Check sheet for the modelled part. Datum: model origin and axes. Units: mm. Face numbers are marked on the shaded views. A direction names the side the tool comes from. Give positions to 0.01 mm unless a question says otherwise; leave off trailing zeros. Order: outer loops, then holes, each group sorted by start corner. A loop starts at its lowest first (then second) coordinate and runs counter-clockwise, first axis right, second up. Notation, with made-up numbers: (44, -22) -> (61, -22) arc R29 ccw to (61, 10) -> close; hole circle Ø4 at (46.5, 51). An arc over 180 degrees is marked (long way). Answer in a Markdown table with one row per item. Add a question column.
(1) Thickness scan on L1, parallel to Z at x = -22, y = 269; L2, parallel to X at y = 117.5, z = -7.5; L3, parallel to Z at x = 4, y = 8. Record the ranges inside material, lowest first. Write a range as [from, to].
(2) Cross-section at D-D (y = 2). Record the cut outline in (x, z).
(3) Cross-section at B-B (x = 5). Record the cut outline in (y, z).
(4) Cross-section at C-C (y = 521.5). Record the cut outline in (x, z), then the cut area to 3 significant figures.
(5) Release check for a two-part mould opening along Z. For the marked faces 1, 2, 3 and 4 record: released by +Z, released by -Z, zero draft, split by the parting line, or undercut.
(6) Cross-section at A-A (z = 10). Record the cut outline in (x, y).
(7) Set-up check for the marked faces 5 and 6: record each of +Z, -Z, +X, -X, +Y, -Y from which the full face is reachable in a straight line by a thin tool's end or side.
(8) Go/stop test with a flat-tipped pin: pin 1 (1.5 mm diameter, centred on x = 29, y = -6.5, fed in from -Z). Record where the tip stops, or that it passes through.
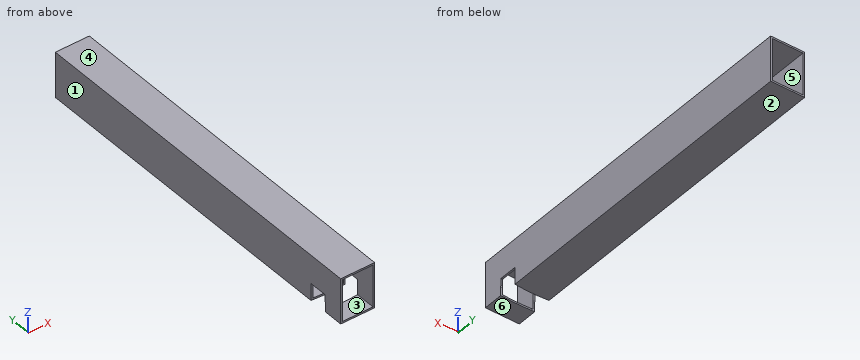
```python
from build123d import *

# Parameters (mm, degrees)
F0_W          = 60
F0_H          = 80
F0_W_2        = 54
F0_H_2        = 74
F1_DEPTH      = 600
F1_DEPTH_BACK = 50
F3_DEPTH      = 30.001
F3_DEPTH_BACK = 30.001
F5_DEPTH      = 30


with BuildPart() as f1:
    # F0 (on Front) → F1 (new body, two sides)
    with BuildSketch(Plane.XZ) as f1_sk:
        with Locations((0, 10)):
            Rectangle(F0_W, F0_H)
        with Locations((0, 10)):
            Rectangle(F0_W_2, F0_H_2, mode=Mode.SUBTRACT)
    extrude(amount=-F1_DEPTH)
    extrude(f1_sk.sketch, amount=F1_DEPTH_BACK)

    # F2 (on Right) → F3 (cut, two sides)
    with BuildSketch(Plane.YZ) as f3_sk:
        with BuildLine():
            Line((15, -30), (15, -15))
            ThreePointArc((15, -15), (0, 0), (-15, -15))
            Line((-15, -15), (-15, -30))
            Line((-15, -30), (15, -30))
        make_face()
    extrude(amount=-F3_DEPTH, mode=Mode.SUBTRACT)
    extrude(f3_sk.sketch, amount=F3_DEPTH_BACK, mode=Mode.SUBTRACT)

    # F4 (on face) → F5 (cut)
    with BuildSketch(Plane(origin=(0, 0, -30), x_dir=(1, 0, 0), z_dir=(0, 0, -1))):
        with BuildLine():
            Line((30, -17.67809667), (30, 14.5012520842))
            ThreePointArc((30, 14.5012520842), (0, 16), (-30, 14.5012520842))
            Line((-30, 14.5012520842), (-30, -17.67809667))
            ThreePointArc((-30, -17.67809667), (0, -16), (30, -17.67809667))
        make_face()
    extrude(amount=-F5_DEPTH, mode=Mode.SUBTRACT)


solid = f1.part
```
Answer below:
| question | item | result |
|---|---|---|
| 1 | L1 | z = [-30, -27], [47, 50] |
| 1 | L2 | x = [-30, -27], [27, 30] |
| 1 | L3 | z = [47, 50] |
| 2 | outline | (-30, 0) -> (-27, 0) -> (-27, 47) -> (27, 47) -> (27, 0) -> (30, 0) -> (30, 50) -> (-30, 50) -> close |
| 3 | outline | (-50, -30) -> (-15.96, -30) -> (-15.96, -27) -> (-50, -27) -> close; (-50, 47) -> (600, 47) -> (600, 50) -> (-50, 50) -> close; (16.05, -30) -> (600, -30) -> (600, -27) -> (16.05, -27) -> close |
| 4 | outline | (-30, -30) -> (30, -30) -> (30, 50) -> (-30, 50) -> close; hole (-27, -27) -> (27, -27) -> (27, 47) -> (-27, 47) -> close |
| 4 | area | 804 mm² |
| 5 | face 1 | zero draft |
| 5 | face 2 | released by -Z |
| 5 | face 3 | undercut |
| 5 | face 4 | released by +Z |
| 6 | outline | (-30, -50) -> (-27, -50) -> (-27, 600) -> (-30, 600) -> close; (27, -50) -> (30, -50) -> (30, 600) -> (27, 600) -> close |
| 7 | face 5 | +Y, -Y |
| 7 | face 6 | -Z, +X, -X, +Y, -Y |
| 8 | pin 1 | stops at z = 0 |
